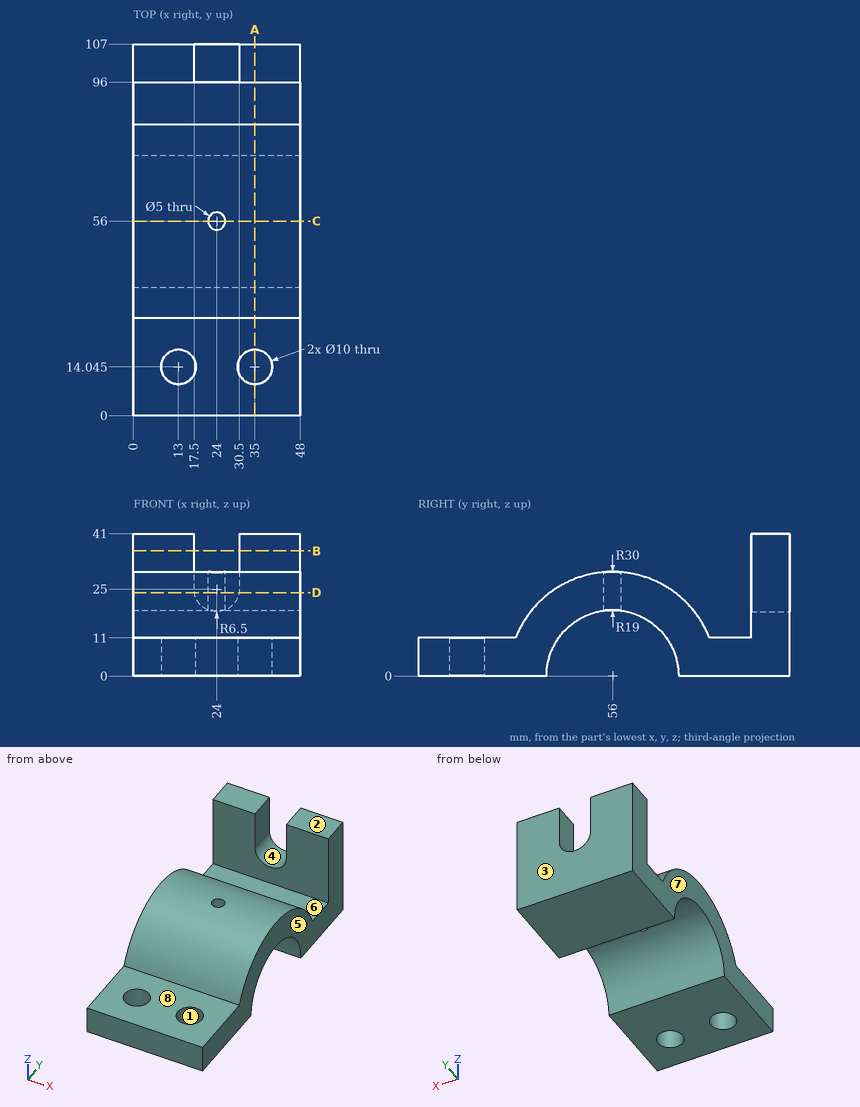
For this review, use the dimensioned drawing (mm, ordinates from the lowest corner) and the shaded views. A direction names the side the tool comes from. Coordinates: 2 decimals unless noted, no trailing zeros. Loops run counter-clockwise (first coordinate to the right, second up) from the corner with the lowest first, then second, coordinate; pieces in that order, holes last. Notation, with made-up numbers: (-15, 30.5) -> (-6, 30.5) arc R16 ccw to (-6, 50.5) -> close; hole circle Ø8 at (76, 4). An arc over 180 degrees is marked (long way). Use a Markdown table: item, result. Add a question column.
Item 1: Machinability: for the marked faces 4, 5, 6, 7 and 8, which of the approach directions +Z, -Z, +X, -X, +Y, -Y give a long, thin tool a straight path to every point of the face, cutting with its end or side? Answer none if there is none.
Item 2: We need section A-A, the plane x = 35. Write out the cut boundary in (y, z) (1 decimal), and give its area (3 significant figures).
Item 3: Wall thickness on L1, parallel to X at y = 16, z = 3.5; L2, parallel to X at y = 56, z = 26.5; L3, parallel to Y at x = 13, z = 5.5 (1 decimal): over which ranges is each line inside the solid? List them lowest first. Write a range as from..to.
Item 4: We need section C-C, the plane y = 56. Write out the cut boundary in (x, z).
Item 5: We need section B-B, the plane z = 36. Write out the cut boundary in (x, y), and give its area (3 significant figures).
Item 6: Clearance check with flat-ended pins moving along their axes: P1, Ø1.5, axis at x = 14.5, y = 62, coming from the -Z side; P2, Ø8.5, axis at x = 19, y = 14.5, coming from the +Z side; P3, Ø9, axis at x = 21.5, z = 25, coming from the -Y side. State where each tip first meets the part, or that it passes through.
Item 7: The part is to be moulded in two halves that separate along Y. For the marked faces 1, 2 and 3, say which applies: +Y half, -Y half, draft (parallel to the pull), parting line (faces both ways), or undercut.
Item 8: We need section D-D, the plane z = 24. Write out the cut boundary in (x, y), and give its area (4 significant figures).
Numbers:
| question | item | result |
|---|---|---|
| 1 | face 4 | +Z, +Y |
| 1 | face 5 | +Z, -Z, +X, +Y, -Y |
| 1 | face 6 | +Z, +X, -X |
| 1 | face 7 | +Z, -Z, -X, +Y, -Y |
| 1 | face 8 | +Z, +X, -X, -Y |
| 2 | outline | (0, 0) -> (9, 0) -> (9, 11) -> (0, 11) -> close; (19, 0) -> (37, 0) arc R19 cw to (75, 0) -> (107, 0) -> (107, 41) -> (96, 41) -> (96, 11) -> (83.9, 11) arc R30 ccw to (28.1, 11) -> (19, 11) -> close |
| 2 | area | 1,600 mm^2 |
| 3 | L1 | x = 0..8.4, 17.6..30.4, 39.6..48 |
| 3 | L2 | x = 0..21.5, 26.5..48 |
| 3 | L3 | y = 0..9, 19..37.8, 74.2..107 |
| 4 | outline | (0, 19) -> (21.5, 19) -> (21.5, 30) -> (0, 30) -> close; (26.5, 19) -> (48, 19) -> (48, 30) -> (26.5, 30) -> close |
| 5 | outline | (0, 96) -> (17.5, 96) -> (17.5, 107) -> (0, 107) -> close; (30.5, 96) -> (48, 96) -> (48, 107) -> (30.5, 107) -> close |
| 5 | area | 385 mm^2 |
| 6 | P1 | stops at z = 17.76 |
| 6 | P2 | stops at z = 11 |
| 6 | P3 | stops at y = 34.1 |
| 7 | face 1 | undercut |
| 7 | face 2 | draft |
| 7 | face 3 | +Y half |
| 8 | outline | (0, 38) -> (48, 38) -> (48, 74) -> (0, 74) -> close; (0, 96) -> (17.58, 96) -> (17.58, 107) -> (0, 107) -> close; (30.42, 96) -> (48, 96) -> (48, 107) -> (30.42, 107) -> close; hole circle Ø5 at (24, 56) |
| 8 | area | 2,095 mm^2 |
